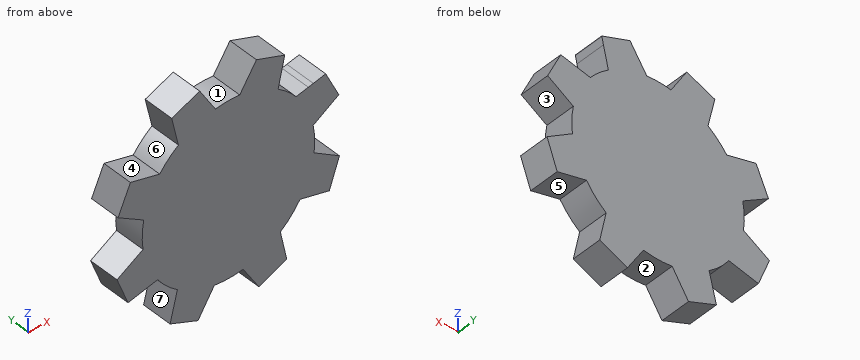
from build123d import *

# Parameters (mm, degrees)
F0_R     = 10.5352835121
F1_DEPTH = 10
F2_R     = 10.5352835121
F4_DEPTH = 10


with BuildPart() as f1:
    # F0 (on Front) → F1 (new body)
    with BuildSketch(Plane.XZ):
        with BuildLine():
            ThreePointArc((27.7799711237, -2.671018116), (28.1744534053, 0.0443174404), (28.3063539053, 2.7849862844))
            ThreePointArc((28.3063539053, 2.7849862844), (28.0187327637, 6.8265473039), (27.1616666974, 10.7866456806))
            ThreePointArc((27.1616666974, 10.7866456806), (25.7257105116, 14.6441244213), (23.7497903046, 18.2549209731))
            ThreePointArc((23.7497903046, 18.2549209731), (19.361792777, 23.5343393933), (13.840033917, 27.6131823971))
            ThreePointArc((13.840033917, 27.6131823971), (10.2093532061, 29.3452118388), (6.3712126192, 30.5495561611))
            ThreePointArc((6.3712126192, 30.5495561611), (-0.2384881302, 31.3241628205), (-6.8478808449, 30.5469322125))
            ThreePointArc((-6.8478808449, 30.5469322125), (-10.969919952, 29.2273648204), (-14.8450148239, 27.2996448624))
            ThreePointArc((-14.8450148239, 27.2996448624), (-20.0530528407, 23.3189368581), (-24.2154366907, 18.2549209731))
            ThreePointArc((-24.2154366907, 18.2549209731), (-26.4192319908, 14.132083875), (-27.9203856002, 9.7047780009))
            ThreePointArc((-27.9203856002, 9.7047780009), (-28.7702301145, 3.1028473381), (-28.0676480896, -3.5163748724))
            ThreePointArc((-28.0676480896, -3.5163748724), (-26.6541111331, -8.0039049024), (-24.5224980596, -12.1982151202))
            ThreePointArc((-24.5224980596, -12.1982151202), (-20.3786644673, -17.4296051981), (-15.133187526, -21.555592431))
            ThreePointArc((-15.133187526, -21.555592431), (-10.8750457734, -23.6957185401), (-6.3201455519, -25.0974299658))
            ThreePointArc((-6.3201455519, -25.0974299658), (0.4193178956, -25.7467388904), (7.122076621, -24.7901851235))
            ThreePointArc((7.122076621, -24.7901851235), (11.5833738131, -23.1931221487), (15.7189210631, -20.8798924315))
            ThreePointArc((15.7189210631, -20.8798924315), (20.7808637814, -16.5258808424), (24.6926258312, -11.1148921464))
            ThreePointArc((24.6926258312, -11.1148921464), (26.5708921122, -7.0152930628), (27.7799711237, -2.671018116))
        make_face()
        with Locations((-0.2328231931, 2.7849862844)):
            Circle(F0_R, mode=Mode.SUBTRACT)
        with BuildLine():
            ThreePointArc((-24.2154366907, 18.2549209731), (-20.0530528407, 23.3189368581), (-14.8450148239, 27.2996448624))
            Line((-14.8450148239, 27.2996448624), (-22.8760878199, 33.2579891401))
            Line((-22.8760878199, 33.2579891401), (-30.0983452841, 26.3414150516))
            Line((-30.0983452841, 26.3414150516), (-24.2154366907, 18.2549209731))
        make_face()
        with BuildLine():
            ThreePointArc((-28.0676480896, -3.5163748724), (-28.7702301145, 3.1028473381), (-27.9203856002, 9.7047780009))
            Line((-27.9203856002, 9.7047780009), (-37.8038170807, 8.1823515919))
            Line((-37.8038170807, 8.1823515919), (-37.9221875331, -1.8169478053))
            Line((-37.9221875331, -1.8169478053), (-28.0676480896, -3.5163748724))
        make_face()
        with BuildLine():
            Line((-23.298226533, -27.3289916042), (-15.133187526, -21.555592431))
            ThreePointArc((-15.133187526, -21.555592431), (-20.3786644673, -17.4296051981), (-24.5224980596, -12.1982151202))
            Line((-24.5224980596, -12.1982151202), (-30.3999287678, -20.2886915134))
            Line((-30.3999287678, -20.2886915134), (-23.298226533, -27.3289916042))
        make_face()
        with BuildLine():
            Line((5.3968944368, -34.640248394), (7.122076621, -24.7901851235))
            ThreePointArc((7.122076621, -24.7901851235), (0.4193178956, -25.7467388904), (-6.3201455519, -25.0974299658))
            Line((-6.3201455519, -25.0974299658), (-4.5983661602, -34.9480886101))
            Line((-4.5983661602, -34.9480886101), (5.3968944368, -34.640248394))
        make_face()
        with BuildLine():
            Line((30.4305433725, -19.3049044961), (24.6926258312, -11.1148921464))
            ThreePointArc((24.6926258312, -11.1148921464), (20.7808637814, -16.5258808424), (15.7189210631, -20.8798924315))
            Line((15.7189210631, -20.8798924315), (23.7909685899, -26.7826078003))
            Line((23.7909685899, -26.7826078003), (30.4305433725, -19.3049044961))
        make_face()
        with BuildLine():
            ThreePointArc((27.1616666974, 10.7866456806), (28.0187327637, 6.8265473039), (28.3063539053, 2.7849862844))
            ThreePointArc((28.3063539053, 2.7849862844), (28.1744534053, 0.0443174404), (27.7799711237, -2.671018116))
            Line((27.7799711237, -2.671018116), (37.6319898333, -0.9570381434))
            Line((37.6319898333, -0.9570381434), (37.004966841, 9.0232846052))
            Line((37.004966841, 9.0232846052), (27.1616666974, 10.7866456806))
        make_face()
        with BuildLine():
            ThreePointArc((13.840033917, 27.6131823971), (19.361792777, 23.5343393933), (23.7497903046, 18.2549209731))
            Line((23.7497903046, 18.2549209731), (29.4473420196, 26.4730658036))
            Line((29.4473420196, 26.4730658036), (22.097377097, 33.2537748843))
            Line((22.097377097, 33.2537748843), (13.840033917, 27.6131823971))
        make_face()
        with BuildLine():
            ThreePointArc((-6.8478808449, 30.5469322125), (-0.2384881302, 31.3241628205), (6.3712126192, 30.5495561611))
            Line((6.3712126192, 30.5495561611), (4.7536209633, 40.4178588133))
            Line((4.7536209633, 40.4178588133), (-5.2463790367, 40.4178588133))
            Line((-5.2463790367, 40.4178588133), (-6.8478808449, 30.5469322125))
        make_face()
    extrude(amount=F1_DEPTH)


with BuildPart() as f4:
    # F2 (on face) → F4 (new body)
    with BuildSketch(Plane.XZ.offset(10)):
        with BuildLine():
            Line((6.0436061547, -23.2930321543), (3.9465958394, -13.5153766205))
            ThreePointArc((3.9465958394, -13.5153766205), (7.4913970999, -10.2975314551), (10.4484246026, -6.5324110277))
            Line((10.4484246026, -6.5324110277), (20.145561814, -8.9748544564))
            Line((20.145561814, -8.9748544564), (23.4940421304, 0.4478669961))
            Line((23.4940421304, 0.4478669961), (15.1021918552, 5.8863271605))
            ThreePointArc((15.1021918552, 5.8863271605), (15.3048791393, 10.3911595364), (14.795466022, 14.8716835175))
            Line((14.795466022, 14.8716835175), (23.2844256021, 20.1572833176))
            Line((23.2844256021, 20.1572833176), (18.9582119637, 29.1730403882))
            Line((18.9582119637, 29.1730403882), (14.8616590906, 28.3110547216))
            Line((14.8616590906, 28.3110547216), (13.840033917, 27.6131823971))
            ThreePointArc((13.840033917, 27.6131823971), (13.5236804737, 27.7898505375), (13.2051095461, 27.9624880101))
            Line((13.2051095461, 27.9624880101), (9.1724991444, 27.1139569468))
            ThreePointArc((9.1724991444, 27.1139569468), (6.3915510384, 30.1271942866), (3.2074944908, 32.7108071709))
            Line((3.2074944908, 32.7108071709), (4.8336037454, 39.9299147155))
            Line((4.8336037454, 39.9299147155), (4.7536209633, 40.4178588133))
            Line((4.7536209633, 40.4178588133), (-5.2463790367, 40.4178588133))
            Line((-5.2463790367, 40.4178588133), (-6.8478808449, 30.5469322125))
            ThreePointArc((-6.8478808449, 30.5469322125), (-10.969919952, 29.2273648204), (-14.8450148239, 27.2996448624))
            Line((-14.8450148239, 27.2996448624), (-22.8760878199, 33.2579891401))
            Line((-22.8760878199, 33.2579891401), (-30.0983452841, 26.3414150516))
            Line((-30.0983452841, 26.3414150516), (-24.2154366907, 18.2549209731))
            ThreePointArc((-24.2154366907, 18.2549209731), (-26.4192319908, 14.132083875), (-27.9203856002, 9.7047780009))
            Line((-27.9203856002, 9.7047780009), (-37.8038170807, 8.1823515919))
            Line((-37.8038170807, 8.1823515919), (-37.9221875331, -1.8169478053))
            Line((-37.9221875331, -1.8169478053), (-28.0676480896, -3.5163748724))
            ThreePointArc((-28.0676480896, -3.5163748724), (-26.6541111331, -8.0039049024), (-24.5224980596, -12.1982151202))
            Line((-24.5224980596, -12.1982151202), (-30.3999287678, -20.2886915134))
            Line((-30.3999287678, -20.2886915134), (-23.298226533, -27.3289916042))
            Line((-23.298226533, -27.3289916042), (-17.896228959, -18.9136233882))
            ThreePointArc((-17.896228959, -18.9136233882), (-13.1442498661, -19.2768415054), (-8.3980860704, -18.8442193547))
            Line((-8.3980860704, -18.8442193547), (-3.10576712, -27.3289916042))
            Line((-3.10576712, -27.3289916042), (6.0436061547, -23.2930321543))
        make_face()
        with Locations((-0.2328231931, 2.7849862844)):
            Circle(F2_R, mode=Mode.SUBTRACT)
        with BuildLine():
            Line((-32.5227899129, -23.4679774305), (-23.298226533, -27.3289916042))
            Line((-23.298226533, -27.3289916042), (-30.3999287678, -20.2886915134))
            Line((-30.3999287678, -20.2886915134), (-24.5224980596, -12.1982151202))
            ThreePointArc((-24.5224980596, -12.1982151202), (-26.6541111331, -8.0039049024), (-28.0676480896, -3.5163748724))
            Line((-28.0676480896, -3.5163748724), (-37.9221875331, -1.8169478053))
            Line((-37.9221875331, -1.8169478053), (-37.8038170807, 8.1823515919))
            Line((-37.8038170807, 8.1823515919), (-27.9203856002, 9.7047780009))
            ThreePointArc((-27.9203856002, 9.7047780009), (-26.4192319908, 14.132083875), (-24.2154366907, 18.2549209731))
            Line((-24.2154366907, 18.2549209731), (-30.0983452841, 26.3414150516))
            Line((-30.0983452841, 26.3414150516), (-22.8760878199, 33.2579891401))
            Line((-22.8760878199, 33.2579891401), (-14.8450148239, 27.2996448624))
            ThreePointArc((-14.8450148239, 27.2996448624), (-10.969919952, 29.2273648204), (-6.8478808449, 30.5469322125))
            Line((-6.8478808449, 30.5469322125), (-5.2463790367, 40.4178588133))
            Line((-5.2463790367, 40.4178588133), (4.7536209633, 40.4178588133))
            Line((4.7536209633, 40.4178588133), (4.8336037454, 39.9299147155))
            Line((4.8336037454, 39.9299147155), (5.3773912439, 42.3440578129))
            Line((5.3773912439, 42.3440578129), (5.4049445449, 42.4663806169))
            Line((5.4049445449, 42.4663806169), (-3.952331747, 45.9936147169))
            Line((-3.952331747, 45.9936147169), (-9.4897229207, 37.6667125925))
            ThreePointArc((-9.4897229207, 37.6667125925), (-13.5099465153, 37.8436589686), (-17.5150931781, 37.4533924182))
            Line((-17.5150931781, 37.4533924182), (-22.7174583218, 45.9936147169))
            Line((-22.7174583218, 45.9936147169), (-31.9867384026, 42.2412225755))
            Line((-31.9867384026, 42.2412225755), (-29.767256543, 32.4906379635))
            ThreePointArc((-29.767256543, 32.4906379635), (-33.0929366105, 29.720743274), (-35.9615144592, 26.4797980987))
            Line((-35.9615144592, 26.4797980987), (-45.6415453785, 28.9891807718))
            Line((-45.6415453785, 28.9891807718), (-49.7406882781, 19.867940314))
            Line((-49.7406882781, 19.867940314), (-41.2532858507, 14.5798404628))
            ThreePointArc((-41.2532858507, 14.5798404628), (-41.7489952856, 9.9313168673), (-41.4791578337, 5.2642313516))
            Line((-41.4791578337, 5.2642313516), (-50.0691131996, 0.1444006111))
            Line((-50.0691131996, 0.1444006111), (-46.4267048395, -9.168647297))
            Line((-46.4267048395, -9.168647297), (-36.6545645454, -7.0460842067))
            ThreePointArc((-36.6545645454, -7.0460842067), (-33.660420308, -10.6752869818), (-30.1106987778, -13.7632457827))
            Line((-30.1106987778, -13.7632457827), (-32.5227899129, -23.4679774305))
        make_face()
        with BuildLine():
            Line((13.840033917, 27.6131823971), (14.8616590906, 28.3110547216))
            Line((14.8616590906, 28.3110547216), (13.2051095461, 27.9624880101))
            ThreePointArc((13.2051095461, 27.9624880101), (13.5236804737, 27.7898505375), (13.840033917, 27.6131823971))
        make_face()
        with Locations((-0.2328231931, 2.7849862844)):
            Circle(F2_R)
    extrude(amount=F4_DEPTH)


solid = f4.part
Read the model definition and answer for the solid it produces. Units are mm, in the model's axes. Face numbers are marked on the shaded views. A direction names the side the tool comes from. Give positions to 0.01 mm unless a question says otherwise; leave off trailing zeros. Loops run counter-clockwise (first coordinate to the right, second up) from the corner with the lowest first, then second, coordinate; pieces in that order, holes last. Notation, with made-up numbers: M 18.25,1.25 L 25.25,1.25 A7 cw 25.25,7.25 Z; hole C -12.75,16 d8. An arc over 180 degrees is marked long. Write each question's results on one line, items separated by ' | '.
1. Straight lines are drawn through the part: line 1 (Z direction, x = -12.5, y = -17.5); line 2 (X direction, y = -17, z = -22); line 3 (X direction, y = -14, z = 14.5). For each, find the intervals that lie inside material, in ascending order. Write a range as [from, to].
Values:
line 1: z = [-19.26, 37.85] | line 2: x = [-32.16, -19.88], [-6.43, 5.77] | line 3: x = [-41.27, 14.87]
2. Section C-C on x = -5 is taken. Give the vertices of the cut face in (y, z), plus the area to 3 significant figures.
Values:
outline: M -20,-24.29 L -10,-24.29 L -10,44.42 L -20,44.42 Z | area: 687 mm^2
3. Section B-B on z = -12 is taken. Give the vertices of the cut face in (x, y), plus the area to 3 significant figures.
Values:
outline: M -32.28,-20 L 5.77,-20 L 5.77,-10 L -32.28,-10 Z | area: 380 mm^2
4. The mould has two halves that part along Z. Classify the marked faces 1, 2 and 3: pulls with the +Z half, pulls with the -Z half, needs draft (parallel to the pull), parting line crosses it, or undercut.
Values:
face 1: pulls with the +Z half | face 2: pulls with the -Z half | face 3: undercut
5. Given pin 1 (12 mm diameter, centred on x = -39.5, z = 37.5, fed in from -Y); pin 2 (3 mm diameter, centred on x = -9, y = -11, fed in from -Z), each flat-ended and moving along its own axis, determine where each tip first touches the part or whether it passes through.
Values:
pin 1: passes through | pin 2: stops at z = -20.28
6. Section A-A on x = 17 is taken. Give the vertices of the cut face in (y, z).
Values:
outline: M -20,-8.18 L -10,-8.18 L -10,4.66 L -20,4.66 Z; M -20,16.24 L -10,16.24 L -10,28.76 L -20,28.76 Z
7. A tool of negligible diameter and unlimited length cuts with its end or side. For the marked faces 4, 5, 6 and 7, from which of +Z, -Z, +X, -X, +Y, -Y can it reach the whole face along a straight path? Write none if from no direction.
Values:
face 4: +Z, +Y, -Y | face 5: -Z, +Y, -Y | face 6: +Y, -Y | face 7: -X, +Y, -Y
